```python
from build123d import *

# Parameters (mm, degrees)
MODEL_R             = 3.175
BOSS_EXTRUDE1_DEPTH = 3.048
BOSS_EXTRUDE2_START = -3.048
SKETCH2_R           = 5.715
SKETCH2_R_2         = 1.4224
BOSS_EXTRUDE2_DEPTH = 3.048


with BuildPart() as part:
    # Model → Boss-Extrude1 (new body)
    with BuildSketch(Plane.XY):
        with BuildLine():
            ThreePointArc((-0.616026415, 14.286925194), (-1.042592722, 15.739677645), (-1.800954663, 17.050149187))
            ThreePointArc((-1.800954663, 17.050149187), (-2.148838289, 17.009806554), (-2.495825317, 16.962366609))
            ThreePointArc((-2.495825317, 16.962366609), (-2.904460903, 15.504468994), (-2.956341002, 13.991274707))
            ThreePointArc((-2.956341002, 13.991274707), (-3.556315124, 13.850932921), (-4.149686627, 13.684875627))
            ThreePointArc((-4.149686627, 13.684875627), (-4.924136412, 14.985904462), (-5.984574038, 16.066608185))
            ThreePointArc((-5.984574038, 16.066608185), (-6.311495456, 15.941017851), (-6.635783413, 15.808776154))
            ThreePointArc((-6.635783413, 15.808776154), (-6.669016568, 14.295057536), (-6.342950641, 12.816500973))
            ThreePointArc((-6.342950641, 12.816500973), (-6.88917389, 12.531360786), (-7.422606766, 12.222954996))
            ThreePointArc((-7.422606766, 12.222954996), (-8.496278501, 13.290511787), (-9.792160616, 14.073543103))
            ThreePointArc((-9.792160616, 14.073543103), (-10.077578151, 13.870596369), (-10.358790833, 13.661862153))
            ThreePointArc((-10.358790833, 13.661862153), (-10.014533394, 12.187435039), (-9.331009364, 10.836419348))
            ThreePointArc((-9.331009364, 10.836419348), (-9.789160524, 10.424397166), (-10.229137224, 9.993021149))
            ThreePointArc((-10.229137224, 9.993021149), (-11.534568165, 10.760027378), (-12.98446973, 11.196185548))
            ThreePointArc((-12.98446973, 11.196185548), (-13.210449547, 10.928634304), (-13.430917328, 10.656523107))
            ThreePointArc((-13.430917328, 10.656523107), (-12.730800257, 9.314031176), (-11.732766451, 8.175445642))
            ThreePointArc((-11.732766451, 8.175445642), (-12.0740582, 7.662430334), (-12.39293337, 7.135189032))
            ThreePointArc((-12.39293337, 7.135189032), (-13.84809849, 7.553450876), (-15.360916858, 7.615330478))
            ThreePointArc((-15.360916858, 7.615330478), (-15.513259815, 7.299985954), (-15.659129891, 6.981595523))
            ThreePointArc((-15.659129891, 6.981595523), (-14.647144119, 5.85539248), (-13.397310672, 5.000778618))
            ThreePointArc((-13.397310672, 5.000778618), (-13.600298394, 4.419004823), (-13.778035935, 3.829026746))
            ThreePointArc((-13.778035935, 3.829026746), (-15.291501858, 3.872263276), (-16.772181085, 3.555976188))
            ThreePointArc((-16.772181085, 3.555976188), (-16.841314914, 3.212652639), (-16.903421733, 2.867988616))
            ThreePointArc((-16.903421733, 2.867988616), (-15.643154047, 2.02883794), (-14.220052592, 1.511894283))
            ThreePointArc((-14.220052592, 1.511894283), (-14.271981822, 0.897916987), (-14.297413829, 0.282272628))
            ThreePointArc((-14.297413829, 0.282272628), (-15.774083925, -0.052232867), (-17.129587491, -0.726813165))
            ThreePointArc((-17.129587491, -0.726813165), (-17.111168259, -1.076543457), (-17.085609422, -1.425824564))
            ThreePointArc((-17.085609422, -1.425824564), (-15.656247076, -1.92519595), (-14.14929631, -2.071987931))
            ThreePointArc((-14.14929631, -2.071987931), (-14.046904143, -2.679590275), (-13.918432631, -3.282217718))
            ThreePointArc((-13.918432631, -3.282217718), (-15.265522286, -3.973447027), (-16.410678917, -4.963934173))
            ThreePointArc((-16.410678917, -4.963934173), (-16.305863972, -5.298096369), (-16.194245434, -5.630047943))
            ThreePointArc((-16.194245434, -5.630047943), (-14.68560052, -5.758262697), (-13.189487703, -5.525679522))
            ThreePointArc((-13.189487703, -5.525679522), (-12.939207816, -6.088729025), (-12.664905121, -6.640474253))
            ThreePointArc((-12.664905121, -6.640474253), (-13.797771739, -7.644994897), (-14.660627033, -8.889152941))
            ThreePointArc((-14.660627033, -8.889152941), (-14.476002283, -9.1867504), (-14.285337446, -9.480514703))
            ThreePointArc((-14.285337446, -9.480514703), (-12.792203675, -9.229516622), (-11.400935076, -8.632172348))
            ThreePointArc((-11.400935076, -8.632172348), (-11.018493474, -9.115290538), (-10.615595045, -9.581485369))
            ThreePointArc((-10.615595045, -9.581485369), (-11.46305645, -10.836179621), (-11.989394033, -12.255833538))
            ThreePointArc((-11.989394033, -12.255833538), (-11.736560131, -12.498167117), (-11.47882917, -12.735285858))
            ThreePointArc((-11.47882917, -12.735285858), (-10.095025626, -12.120846074), (-8.896019768, -11.196274037))
            ThreePointArc((-8.896019768, -11.196274037), (-8.405446665, -11.569104823), (-7.899268091, -11.920456521))
            ThreePointArc((-7.899268091, -11.920456521), (-8.408075165, -13.346487327), (-8.564823313, -14.85243504))
            ThreePointArc((-8.564823313, -14.85243504), (-8.259666742, -15.024278029), (-7.95106384, -15.189852165))
            ThreePointArc((-7.95106384, -15.189852165), (-6.76353999, -14.25057819), (-5.832134822, -13.056872652))
            ThreePointArc((-5.832134822, -13.056872652), (-5.264254728, -13.295989703), (-4.686601071, -13.510421549))
            ThreePointArc((-4.686601071, -13.510421549), (-4.824783595, -15.018186149), (-4.602093245, -16.515803425))
            ThreePointArc((-4.602093245, -16.515803425), (-4.263788115, -16.606358298), (-3.923703928, -16.689984197))
            ThreePointArc((-3.923703928, -16.689984197), (-3.007076261, -15.484894068), (-2.401795395, -14.097059939))
            ThreePointArc((-2.401795395, -14.097059939), (-1.792290307, -14.187438652), (-1.17945767, -14.251477104))
            ThreePointArc((-1.17945767, -14.251477104), (-0.938333127, -15.746237102), (-0.350196733, -17.14142314))
            ThreePointArc((-0.350196733, -17.14142314), (0, -17.145), (0.350196733, -17.14142314))
            ThreePointArc((0.350196733, -17.14142314), (0.938333127, -15.746237102), (1.17945767, -14.251477104))
            ThreePointArc((1.17945767, -14.251477104), (1.792290307, -14.187438652), (2.401795395, -14.097059939))
            ThreePointArc((2.401795395, -14.097059939), (3.007076261, -15.484894068), (3.923703928, -16.689984197))
            ThreePointArc((3.923703928, -16.689984197), (4.263788115, -16.606358298), (4.602093245, -16.515803425))
            ThreePointArc((4.602093245, -16.515803425), (4.824783595, -15.018186149), (4.686601071, -13.510421549))
            ThreePointArc((4.686601071, -13.510421549), (5.264254728, -13.295989704), (5.832134822, -13.056872652))
            ThreePointArc((5.832134822, -13.056872652), (6.76353999, -14.25057819), (7.95106384, -15.189852165))
            ThreePointArc((7.95106384, -15.189852165), (8.259666742, -15.024278029), (8.564823313, -14.85243504))
            ThreePointArc((8.564823313, -14.85243504), (8.408075165, -13.346487327), (7.899268091, -11.920456521))
            ThreePointArc((7.899268091, -11.920456521), (8.405446665, -11.569104823), (8.896019768, -11.196274037))
            ThreePointArc((8.896019768, -11.196274037), (10.095025626, -12.120846074), (11.47882917, -12.735285858))
            ThreePointArc((11.47882917, -12.735285858), (11.736560131, -12.498167117), (11.989394033, -12.255833538))
            ThreePointArc((11.989394033, -12.255833538), (11.46305645, -10.836179621), (10.615595045, -9.581485369))
            ThreePointArc((10.615595045, -9.581485369), (11.018493474, -9.115290538), (11.400935076, -8.632172348))
            ThreePointArc((11.400935076, -8.632172348), (12.792203675, -9.229516622), (14.285337446, -9.480514703))
            ThreePointArc((14.285337446, -9.480514703), (14.476002283, -9.1867504), (14.660627033, -8.889152941))
            ThreePointArc((14.660627033, -8.889152941), (13.797771739, -7.644994897), (12.664905121, -6.640474253))
            ThreePointArc((12.664905121, -6.640474253), (12.939207816, -6.088729025), (13.189487703, -5.525679522))
            ThreePointArc((13.189487703, -5.525679522), (14.68560052, -5.758262697), (16.194245434, -5.630047943))
            ThreePointArc((16.194245434, -5.630047943), (16.305863972, -5.298096369), (16.410678917, -4.963934173))
            ThreePointArc((16.410678917, -4.963934173), (15.265522286, -3.973447027), (13.918432631, -3.282217718))
            ThreePointArc((13.918432631, -3.282217718), (11.018493474, 9.115290538), (-0.616026415, 14.286925194))
        make_face()
        with Locations(Location((0, 0, 0), (0, 0, 180))):
            Circle(MODEL_R, mode=Mode.SUBTRACT)
    extrude(amount=BOSS_EXTRUDE1_DEPTH)

    # Sketch2 → Boss-Extrude2 (add)
    # profile 1 of 2: a face of its own
    with BuildSketch(Plane.XY.offset(3.048).offset(BOSS_EXTRUDE2_START)):
        with BuildLine():
            Line((14.117624536, 37.542772707), (1.307007018, 14.240345947))
            ThreePointArc((1.307007018, 14.240345947), (6.88917389, 12.531360786), (11.323192371, 8.733901452))
            Line((11.323192371, 8.733901452), (24.133809889, 32.036328212))
            ThreePointArc((24.133809889, 32.036328212), (16.372494965, 29.781457783), (14.117624536, 37.542772707))
        make_face()
    # profile 2 of 2: a face of its own
    with BuildSketch(Plane.XY.offset(3.048).offset(BOSS_EXTRUDE2_START)):
        with Locations((19.125717213, 34.789550459)):
            Circle(SKETCH2_R)
        with Locations((19.125717213, 34.789550459)):
            Circle(SKETCH2_R_2, mode=Mode.SUBTRACT)
    extrude(amount=BOSS_EXTRUDE2_DEPTH)


solid = part.part
```
The listing builds one solid part. Answer for the finished solid, in the listing's coordinates (mm). A direction names the side the tool comes from. Give positions to 0.01 mm unless a question says otherwise; leave off trailing zeros. Use one line per item in the form item = value. Start each with the question number.
1) The mould has two halves that part along Y. Classify faces 1 (the face through (-0.944, -15.726, 1.503)), 2 (the face through (12.936, -6.097, 1.503)), 3 (the face through (4, 6, 0)): pulls with the +Y half, pulls with the -Y half, needs draft (parallel to the pull), parting line crosses it, or undercut.
2) A tool of negligible diameter and unlimited length cuts with its end or side. For faces 4 (the face through (10.08, -12.11, 1.5)), 5 (the face through (15.283, -3.985, 1.503)), 6 (the face through (-15.754, -0.045, 1.503)), 7 (the face through (-2.9, 15.53, 1.5)), from which of +Z, -Z, +X, -X, +Y, -Y can it reach the whole face along a straight path? Write none if from no direction.
3) Find section A-A on z = 0.5. Count the separate pieces of the cut face and the enclosed holes in it, plus the area to 3 significant figures.
4) Consider line 1 along X through (y, z) = (15.5, 2.2); line 2 along Y through (x, z) = (-15, 2); line 3 along Y through (x, z) = (0, 0.75) (3 decimals). Determine where each line is inside the solid, lowest interval first. Write a range as from..to.
Geometry results:
q1.face_1 = pulls with the -Y half
q1.face_2 = undercut
q1.face_3 = needs draft
q2.face_4 = +Z, -Z, -Y
q2.face_5 = +Z, -Z, +X
q2.face_6 = +Z, -Z, -X
q2.face_7 = +Z, -Z
q3.separate_pieces = 1
q3.enclosed_holes = 2
q3.area = 1,040 mm2
q4.line_1 = -6.67..-5.37, -2.91..-0.95, 2..15.04
q4.line_2 = -5.76..-3.8, -2.03..0.17, 1.75..3.89, 6.19..7.63
q4.line_3 = -17.145..-3.175, 3.175..14.3
